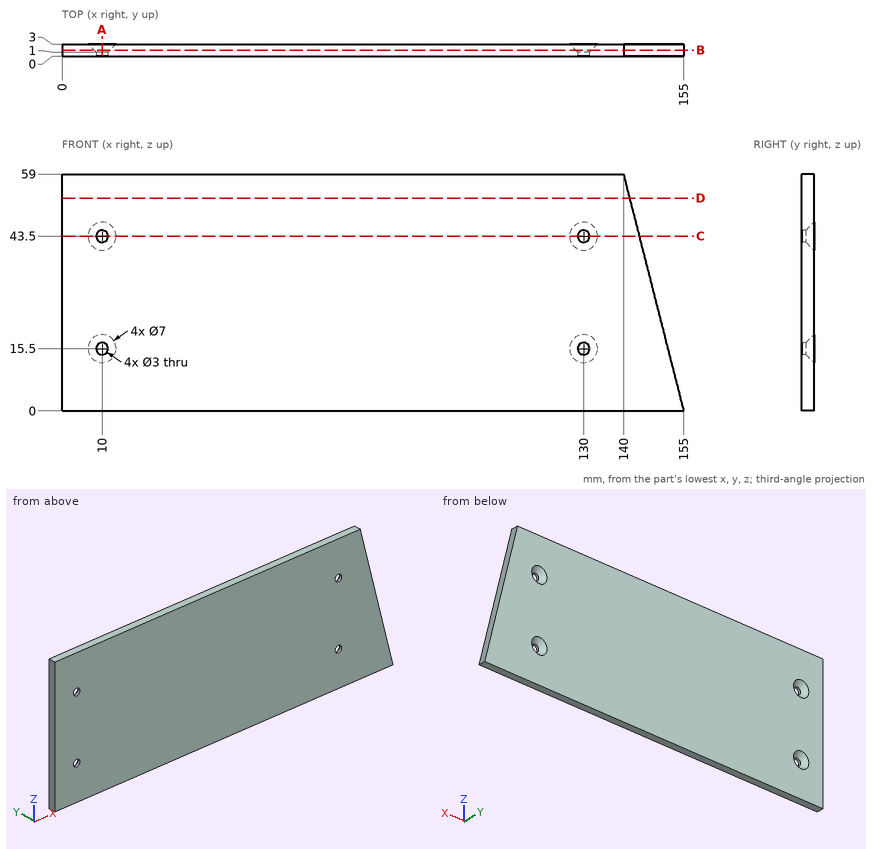
Drawing for the job (mm, zero at the part's lowest x, y, z). Give positions to 0.01 mm unless a question says otherwise; leave off trailing zeros. Loops run counter-clockwise (first coordinate to the right, second up) from the corner with the lowest first, then second, coordinate; pieces in that order, holes last.
Item 1: Slice it at D-D (z = 53). Write the cut outline in (x, y), plus the area to 3 significant figures.
Check values:
outline: (0, 0) - (141.53, 0) - (141.53, 3) - (0, 3) - close
area: 425 mm2
Item 2: Slice it at B-B (y = 1.5). Write the cut outline in (x, z), plus the area to 3 significant figures.
Check values:
outline: (0, 0) - (155, 0) - (140, 59) - (0, 59) - close; hole circle Ø4 at (10, 15.5); hole circle Ø4 at (10, 43.5); hole circle Ø4 at (130, 15.5); hole circle Ø4 at (130, 43.5)
area: 8,650 mm2
Item 3: Slice it at C-C (z = 43.5). Write the cut outline in (x, y).
Check values:
outline: (0, 0) - (8.5, 0) - (8.5, 1) - (6.5, 3) - (0, 3) - close; (11.5, 0) - (128.5, 0) - (128.5, 1) - (126.5, 3) - (13.5, 3) - (11.5, 1) - close; (131.5, 0) - (143.94, 0) - (143.94, 3) - (133.5, 3) - (131.5, 1) - close
Item 4: Slice it at A-A (x = 10). Write the cut outline in (y, z).
Check values:
outline: (0, 0) - (3, 0) - (3, 12) - (1, 14) - (0, 14) - close; (0, 17) - (1, 17) - (3, 19) - (3, 40) - (1, 42) - (0, 42) - close; (0, 45) - (1, 45) - (3, 47) - (3, 59) - (0, 59) - close
Item 5: Drop flat-ended pins along their axis: P1, Ø3.5, axis at x = 130, z = 43.5, coming from the +Y side; P2, Ø5, axis at x = 10, z = 43.5, coming from the +Y side; P3, Ø2.5, axis at x = 130, z = 15.5, coming from the +Y side; P4, Ø1, axis at y = 2.5, z = 30, coming from the +X side. Give the stop position or say it passes through.
Check values:
P1: stops at y = 1.25
P2: stops at y = 2
P3: passes through
P4: stops at x = 147.5
Item 6: Drill centre lines: line 1 along Z through (x, y) = (130, 0.85); line 2 along X through (y, z) = (2.1, 13.5); line 3 along X through (y, z) = (1.35, 43). Where is each one in solid material? Low to high.
Check values:
line 1: z = 0 to 14, 17 to 42, 45 to 59
line 2: x = 0 to 8.34, 11.66 to 128.34, 131.66 to 151.57
line 3: x = 0 to 8.22, 11.78 to 128.22, 131.78 to 144.07
